Here's how the part is built. I have some questions about the finished solid (model axes, mm). A direction names the side the tool comes from. Give positions to 0.01 mm unless a question says otherwise; leave off trailing zeros. Loops run counter-clockwise (first coordinate to the right, second up) from the corner with the lowest first, then second, coordinate; pieces in that order, holes last. Notation, with made-up numbers: (31.25, 26.5) -> (38.25, 26.5) arc R31 ccw to (38.25, 64.5) -> close; hole circle Ø4 at (9, 20). An arc over 180 degrees is marked (long way). Answer in a Markdown table with one row per item. Add a question column.
Item 1: If we section it at B-B (z = -8): Write out the boundary of the cut face in (x, y).
Item 2: If I drill on line 1 (X direction, y = 3.75, z = 0); line 2 (X direction, y = 4.75, z = 0.75); line 3 (Z direction, x = -4.75, y = 5), over which ranges is the centre line in solid material (lowest first)?
Item 3: For P1, Ø1.6, axis at x = 2.5, z = 0, coming from the +Y side; P2, Ø9, axis at x = -2, z = 1.5, coming from the -Y side; P3, Ø2.5, axis at x = 0, z = 8, coming from the +Y side; P4, Ø2, axis at x = 2.5, z = -1, coming from the -Y side, each with a flat end and sliding along its axis, tell me the tip position at first contact or that it passes through.
Item 4: Which directions (+Z, -Z, +X, -X, +Y, -Y) give clear straight access to the entire face, cutting with the end or side of a thin tool? Please do faces 5 (the face through (-5, 0, 0)), 6 (the face through (0, 5.5, 0)), 7 (the face through (1.802, 7.965, 5.723)).
Item 5: We'd pull the mould along Z, two halves only. Please class faces 1 (the face through (0, 10.5, 0)), 2 (the face through (-10.74, 2.71, -2.38)), 3 (the face through (4.68, 2.71, 5.44)), 4 (the face through (-4.665, 2.712, 5.527)): released by +Z, released by -Z, zero draft, split by the parting line, or undercut.
Item 6: If we section it at C-C (x = 8): Write out the boundary of the cut face in (y, z), then the cut area to 3 significant figures.
Item 7: If we section it at D-D (y = 9.5): Write out the boundary of the cut face in (x, z), then the cut area to 3 significant figures.
Item 8: If we section it at A-A (x = 0): Write out the boundary of the cut face in (y, z).
```python
from build123d import *

# Parameters (mm, degrees)
SKETCH1_R           = 11
SKETCH1_R_2         = 1
BOSS_EXTRUDE1_DEPTH = 5.5
SKETCH2_R           = 4
CUT_EXTRUDE1_DEPTH  = 17.5
SKETCH9_R           = 6
BOSS_EXTRUDE4_DEPTH = 5
SKETCH10_R          = 1
CUT_EXTRUDE6_DEPTH  = 19.768324379


with BuildPart() as part:
    # Sketch1 → Boss-Extrude1 (new body)
    with BuildSketch(Plane(origin=(0, 0, 0), x_dir=(1, 0, 0), z_dir=(0, 1, 0))):
        with Locations(Location((0, 0, 0), (0, 0, 270))):
            Circle(SKETCH1_R)
        with Locations(Location((0, 8, 0), (0, 0, 270))):
            Circle(SKETCH1_R_2, mode=Mode.SUBTRACT)
        with Locations(Location((5.656854249, 5.656854249, 0), (0, 0, 270))):
            Circle(SKETCH1_R_2, mode=Mode.SUBTRACT)
        with Locations(Location((8, 0, 0), (0, 0, 270))):
            Circle(SKETCH1_R_2, mode=Mode.SUBTRACT)
        with Locations(Location((5.656854249, -5.656854249, 0), (0, 0, 270))):
            Circle(SKETCH1_R_2, mode=Mode.SUBTRACT)
        with Locations(Location((0, -8, 0), (0, 0, 270))):
            Circle(SKETCH1_R_2, mode=Mode.SUBTRACT)
        with Locations(Location((-5.656854249, -5.656854249, 0), (0, 0, 270))):
            Circle(SKETCH1_R_2, mode=Mode.SUBTRACT)
        with Locations(Location((-8, 0, 0), (0, 0, 270))):
            Circle(SKETCH1_R_2, mode=Mode.SUBTRACT)
        with Locations(Location((-5.656854249, 5.656854249, 0), (0, 0, 270))):
            Circle(SKETCH1_R_2, mode=Mode.SUBTRACT)
    extrude(amount=BOSS_EXTRUDE1_DEPTH)

    # Sketch2 → Cut-Extrude1 (cut, through all)
    with BuildSketch(Plane(origin=(0, 5.5, 0), x_dir=(1, 0, 0), z_dir=(0, 1, 0))):
        with Locations(Location((0, 0, 0), (0, 0, 270))):
            Circle(SKETCH2_R)
    extrude(amount=-CUT_EXTRUDE1_DEPTH, mode=Mode.SUBTRACT)

    # Sketch9 → Boss-Extrude4 (add)
    with BuildSketch(Plane(origin=(0, 5.5, 0), x_dir=(1, 0, 0), z_dir=(0, 1, 0))):
        with Locations(Location((0, 0, 0), (0, 0, 270))):
            Circle(SKETCH9_R)
    extrude(amount=BOSS_EXTRUDE4_DEPTH)

    # Sketch10 → Cut-Extrude6 (cut, through all)
    with BuildSketch(Plane(origin=(0, 10.5, 0), x_dir=(1, 0, 0), z_dir=(0, 1, 0))):
        with Locations(Location((-2.5, 0, 0), (0, 0, 270))):
            Circle(SKETCH10_R)
        with Locations(Location((2.5, 0, 0), (0, 0, 270))):
            Circle(SKETCH10_R)
    extrude(amount=-CUT_EXTRUDE6_DEPTH, mode=Mode.SUBTRACT)


solid = part.part
```
Recorded:
| question | item | result |
|---|---|---|
| 1 | outline | (-7.55, 0) -> (-1, 0) -> (-1, 5.5) -> (-7.55, 5.5) -> close; (1, 0) -> (7.55, 0) -> (7.55, 5.5) -> (1, 5.5) -> close |
| 2 | line 1 | x = -11 to -9, -7 to -4, 4 to 7, 9 to 11 |
| 2 | line 2 | x = -10.97 to -8.66, -7.34 to -3.93, 3.93 to 7.34, 8.66 to 10.97 |
| 2 | line 3 | z = -9.92 to -6.08, -5.24 to 5.24, 6.08 to 9.92 |
| 3 | P1 | passes through |
| 3 | P2 | stops at y = 0 |
| 3 | P3 | stops at y = 5.5 |
| 3 | P4 | stops at y = 5.5 |
| 4 | face 5 | +Z, -Z, +X, -X, -Y |
| 4 | face 6 | -Y |
| 4 | face 7 | +Y |
| 5 | face 1 | zero draft |
| 5 | face 2 | split by the parting line |
| 5 | face 3 | undercut |
| 5 | face 4 | undercut |
| 6 | outline | (0, -7.55) -> (5.5, -7.55) -> (5.5, -1) -> (0, -1) -> close; (0, 1) -> (5.5, 1) -> (5.5, 7.55) -> (0, 7.55) -> close |
| 6 | area | 72.0 mm^2 |
| 7 | outline | circle Ø12 at (0, 0); hole circle Ø2 at (-2.5, 0); hole circle Ø2 at (2.5, 0) |
| 7 | area | 107 mm^2 |
| 8 | outline | (0, -11) -> (5.5, -11) -> (5.5, -9) -> (0, -9) -> close; (0, -7) -> (5.5, -7) -> (5.5, -6) -> (10.5, -6) -> (10.5, 6) -> (5.5, 6) -> (5.5, 7) -> (0, 7) -> (0, 4) -> (5.5, 4) -> (5.5, -4) -> (0, -4) -> close; (0, 9) -> (5.5, 9) -> (5.5, 11) -> (0, 11) -> close |
